Model file for the job. Use its own axes, mm. Face numbers are marked on the shaded views. A direction names the side the tool comes from. Round coordinates to 2 decimals unless told otherwise and drop trailing zeros. Loops run counter-clockwise (first coordinate to the right, second up) from the corner with the lowest first, then second, coordinate; pieces in that order, holes last.
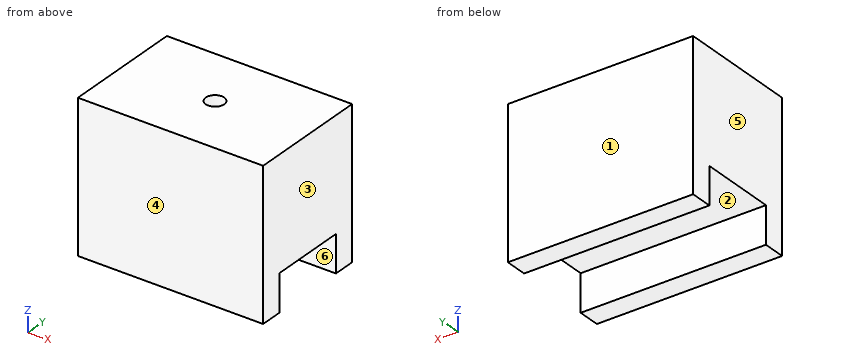
from build123d import *

# Parameters (mm, degrees)
F0_W     = 25
F0_H     = 3
F0_H_2   = 10.5
F1_DEPTH = 20
F2_DEPTH = 5
F3_R     = 1.25
F4_DEPTH = 20.001


with BuildPart() as f1:
    # F0 (on Top) → F1 (new body)
    with BuildSketch(Plane.XY):
        with Locations((0, 6.75)):
            Rectangle(F0_W, F0_H)
        Rectangle(F0_W, F0_H_2)
        with Locations((0, -6.75)):
            Rectangle(F0_W, F0_H)
    extrude(amount=F1_DEPTH)

    # F0 (on Top) → F2 (cut)
    with BuildSketch(Plane.XY):
        Rectangle(F0_W, F0_H_2)
    extrude(amount=F2_DEPTH, mode=Mode.SUBTRACT)

    # F3 (on face) → F4 (cut, through all)
    with BuildSketch(Plane.XY.offset(20)):
        Circle(F3_R)
    extrude(amount=-F4_DEPTH, mode=Mode.SUBTRACT)


solid = f1.part
Q1. Tool access for the marked faces 5 and 6: list every direction of +Z, -Z, +X, -X, +Y, -Y with a clear straight run to the whole face (end or side of a thin tool).
Q2. Slice it at C-C on y = 2.5. Give the cut face in (x, z).
Q3. Pull direction Y, two halves, no side cores. Call the marked faces 1, 2, 3 and 4: pulls with the +Y half, pulls with the -Y half, needs draft (parallel to the pull), parting line crosses it, or undercut.
Q4. Probe line 1 (Y direction, x = 8.5, z = 4); line 2 (Y direction, x = 0, z = 11); line 3 (Z direction, x = -2.5, y = -1.5). List the from-to ranges inside material, lowest first.
Q5. Slice it at A-A on x = 0. Give the cut face in (y, z), plus the area to 3 significant figures.
Q6. Flat gauge pin, fed straight in: P1, Ø5, axis at x = 0.5, y = -2.5, coming from the -Z side. Where does the tip first touch, or does it go through?
Q7. Slice it at B-B on y = 0. Give the cut face in (x, z).
Reply:
1. face 5: +Z, -Z, -X, +Y, -Y
1. face 6: -Z, +X, -X
2. outline: (-12.5, 5) - (12.5, 5) - (12.5, 20) - (-12.5, 20) - close
3. face 1: pulls with the +Y half
3. face 2: undercut
3. face 3: needs draft
3. face 4: pulls with the -Y half
4. line 1: y = -8.25 to -5.25, 5.25 to 8.25
4. line 2: y = -8.25 to -1.25, 1.25 to 8.25
4. line 3: z = 5 to 20
5. outline: (-8.25, 0) - (-5.25, 0) - (-5.25, 5) - (-1.25, 5) - (-1.25, 20) - (-8.25, 20) - close; (1.25, 5) - (5.25, 5) - (5.25, 0) - (8.25, 0) - (8.25, 20) - (1.25, 20) - close
5. area: 240 mm2
6. P1: stops at z = 5
7. outline: (-12.5, 5) - (-1.25, 5) - (-1.25, 20) - (-12.5, 20) - close; (1.25, 5) - (12.5, 5) - (12.5, 20) - (1.25, 20) - close
